Could you check a few things on this model? Use its own coordinates, in mm. Face numbers are marked on the shaded views. Give positions to 0.01 mm unless a question says otherwise; leave off trailing zeros. Loops run counter-clockwise (first coordinate to the right, second up) from the corner with the lowest first, then second, coordinate; pieces in that order, holes last. Notation, with made-up numbers: M -1.5,-23.5 L 22.5,-23.5 A13 ccw 22.5,-17.5 Z; hole C 3.25,-26 d9. An arc over 180 degrees is marked long. Write each question's results on one line, items separated by ' | '. Start each with the question number.
from build123d import *

# Parameters (mm, degrees)
SKETCH1_W           = 190
SKETCH1_H           = 170
BOSS_EXTRUDE1_DEPTH = 10
SKETCH2_W           = 190
SKETCH2_H           = 59
BOSS_EXTRUDE2_DEPTH = 12
SKETCH3_W           = 190
SKETCH3_H           = 59
BOSS_EXTRUDE3_DEPTH = 12
SKETCH4_R           = 5.9
BOSS_EXTRUDE4_DEPTH = 105
SKETCH5_R           = 5.9
BOSS_EXTRUDE5_DEPTH = 105


with BuildPart() as part:
    # Sketch1 → Boss-Extrude1 (new body)
    with BuildSketch(Plane.XY.offset(123)):
        with Locations((300, 300)):
            Rectangle(SKETCH1_W, SKETCH1_H)
    extrude(amount=BOSS_EXTRUDE1_DEPTH)

    # Sketch2 → Boss-Extrude2 (add)
    with BuildSketch(Plane(origin=(0, 385, 0), x_dir=(1, 0, 0), z_dir=(0, 1, 0))):
        with Locations((300, -152.5)):
            Rectangle(SKETCH2_W, SKETCH2_H)
    extrude(amount=BOSS_EXTRUDE2_DEPTH)

    # Sketch3 → Boss-Extrude3 (add)
    with BuildSketch(Plane(origin=(0, 203, 0), x_dir=(1, 0, 0), z_dir=(0, 1, 0))):
        with Locations((300, -152.5)):
            Rectangle(SKETCH3_W, SKETCH3_H)
    extrude(amount=BOSS_EXTRUDE3_DEPTH)

    # Sketch4 → Boss-Extrude4 (add)
    with BuildSketch(Plane(origin=(0, 385, 0), x_dir=(1, 0, 0), z_dir=(0, 1, 0))):
        with Locations(Location((300, -157, 0), (0, 0, 270))):
            Circle(SKETCH4_R)
    extrude(amount=BOSS_EXTRUDE4_DEPTH)

    # Sketch5 → Boss-Extrude5 (add)
    with BuildSketch(Plane(origin=(0, 110, 0), x_dir=(1, 0, 0), z_dir=(0, 1, 0))):
        with Locations(Location((300, -157, 0), (0, 0, 270))):
            Circle(SKETCH5_R)
    extrude(amount=BOSS_EXTRUDE5_DEPTH)


solid = part.part
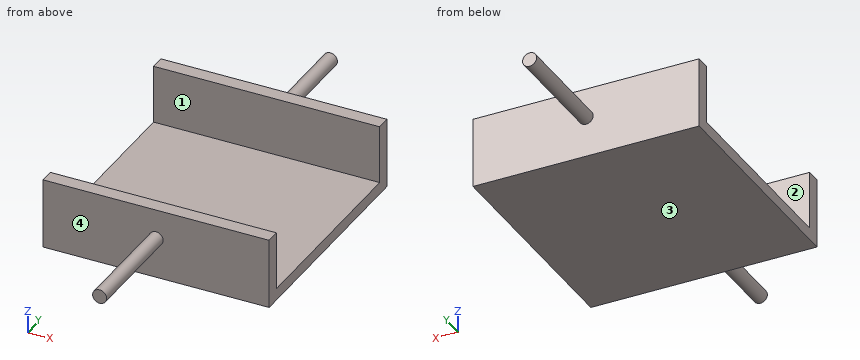
1) If we section it at B-B on x = 271: Write out the boundary of the cut face in (y, z).
2) If we section it at A-A on z = 139: Write out the boundary of the cut face in (x, y), plus the area to 3 significant figures.
3) I'm going to push flat-ended pins straight in: P1, Ø4, axis at x = 235.5, z = 129.5, coming from the -Y side; P2, Ø1, axis at x = 267.5, y = 258, coming from the +Z side; P3, Ø5, axis at y = 399, z = 172.5, coming from the -X side; P4, Ø6, axis at x = 227, y = 400.5, coming from the -Z side. Where does each tip first touch, or does it pass through?
4) Thinking about a two-plate mould opening in Y: for the marked faces 1, 2, 3 and 4, which applies, pulls with the +Y half, pulls with the -Y half, needs draft (parallel to the pull), parting line crosses it, or undercut?
5) If we section it at C-C on z = 157: Write out the boundary of the cut face in (x, y).
6) If we section it at D-D on y = 222: Write out the boundary of the cut face in (x, z), plus the area to 3 significant figures.
7) Please list where these lines run through material, in increasing order: line 1 (Y direction, x = 241.5, z = 174.5); line 2 (Z direction, x = 273.5, y = 248.5); line 3 (Y direction, x = 357, z = 131). Write a range as from..to.
Calculated:
1) outline: M 203,123 L 397,123 L 397,182 L 385,182 L 385,133 L 215,133 L 215,182 L 203,182 Z
2) outline: M 205,203 L 395,203 L 395,215 L 205,215 Z; M 205,385 L 395,385 L 395,397 L 205,397 Z | area: 4,560 mm2
3) P1: stops at y = 203 | P2: stops at z = 133 | P3: stops at x = 205 | P4: passes through
4) face 1: undercut | face 2: undercut | face 3: needs draft | face 4: pulls with the -Y half
5) outline: M 205,203 L 294.1,203 L 294.1,110 L 305.9,110 L 305.9,203 L 395,203 L 395,215 L 205,215 Z; M 205,385 L 395,385 L 395,397 L 305.9,397 L 305.9,490 L 294.1,490 L 294.1,397 L 205,397 Z
6) outline: M 205,123 L 395,123 L 395,133 L 205,133 Z | area: 1,900 mm2
7) line 1: y = 203..215, 385..397 | line 2: z = 123..133 | line 3: y = 203..397
